Read the model definition and answer for the solid it produces. Units are mm, in the model's axes. A direction names the side the tool comes from. Round coordinates to 2 decimals unless told otherwise and drop trailing zeros. Write each loop counter-clockwise with the first axis right and the second up, starting at its lowest first coordinate (ties: lowest second). Pieces come first, ordered by that corner, then holes. Notation, with made-up numbers: (24, 0.25) - (37, 0.25) arc R36 cw to (37, 39.25) - close; hole circle Ø5 at (-27.75, -7). An arc over 180 degrees is marked (long way). Use one line per item in the form item = value. Start each with the question number.
1) The part is cut by section D-D, the plane y = 16.5. Give the vertices of the cut face in (x, z).
2) For a pull along Z with two mould halves and no side action, classify faces 4 (the face through (46, 22, -58)), 5 (the face through (0, 22, -29)), 6 (the face through (66, 32, -10)) as released by +Z, released by -Z, zero draft, split by the parting line, or undercut.
3) The part is cut by section B-B, the plane x = 17. Give the vertices of the cut face in (y, z), plus the area to 3 significant figures.
4) The part is cut by section C-C, the plane y = 4.5. Count the separate pieces of the cut face and the enclosed holes in it, plus the area to 3 significant figures.
5) Consider line 1 along X through (y, z) = (9, -31); line 2 along Z through (x, y) = (49, 12.5); line 3 along X through (y, z) = (13, -33). Determine where each line is inside the solid, lowest interval first. Write a range as from..to.
6) Each of these flat-tipped pins is pushed along its axis until it touches: pin 1 (1.2 mm diameter, centred on x = 67, z = -51.5, fed in from +Y); pin 2 (10 mm diameter, centred on y = 13, z = -51, fed in from -X); pin 3 (2 mm diameter, centred on x = 39, z = -0.5, fed in from +Y); pin 4 (0.6 mm diameter, centred on x = 37, y = 43.5, fed in from +Z). Where does it stop, or does it pass through?
7) The part is cut by section A-A, the plane y = 33. Give the vertices of the cut face in (x, z).
8) For faces 1 (the face through (72, 42, -1)), 2 (the face through (39.714, 16.79, -9.945)), 3 (the face through (94, 22, -29)), determine the directions among +Z, -Z, +X, -X, +Y, -Y from which every point of the face is accessible in a straight line to the end or side of a thin tool.
from build123d import *

# Parameters (mm, degrees)
SKETCH1_W           = 94
SKETCH1_H           = 58
BOSS_EXTRUDE1_DEPTH = 45
SKETCH2_W           = 90
SKETCH2_H           = 54
CUT_EXTRUDE1_DEPTH  = 43
SKETCH6_W           = 92
SKETCH6_H           = 56
CUT_EXTRUDE2_DEPTH  = 2
SKETCH10_R          = 2
SKETCH10_R_2        = 5.056057686
BOSS_EXTRUDE2_DEPTH = 30
SKETCH11_R          = 3.75
CUT_EXTRUDE3_DEPTH  = 2
SKETCH12_W          = 15.1
SKETCH12_H          = 2
CUT_EXTRUDE4_DEPTH  = 11


with BuildPart() as part:
    # Sketch1 → Boss-Extrude1 (new body)
    with BuildSketch(Plane(origin=(0, 0, 0), x_dir=(1, 0, 0), z_dir=(0, 1, 0))):
        with Locations((47, 29)):
            Rectangle(SKETCH1_W, SKETCH1_H)
    extrude(amount=BOSS_EXTRUDE1_DEPTH)

    # Sketch2 → Cut-Extrude1 (cut)
    with BuildSketch(Plane(origin=(0, 45, 0), x_dir=(1, 0, 0), z_dir=(0, 1, 0))):
        with Locations((47, 29)):
            Rectangle(SKETCH2_W, SKETCH2_H)
    extrude(amount=-CUT_EXTRUDE1_DEPTH, mode=Mode.SUBTRACT)

    # Sketch6 → Cut-Extrude2 (cut)
    with BuildSketch(Plane(origin=(0, 43, 0), x_dir=(-1, 0, 0), z_dir=(0, -1, 0))):
        with Locations((-47, 29)):
            Rectangle(SKETCH6_W, SKETCH6_H)
    extrude(amount=CUT_EXTRUDE2_DEPTH, mode=Mode.SUBTRACT)

    # Sketch10 → Boss-Extrude2 (add)
    with BuildSketch(Plane(origin=(0, 2, 0), x_dir=(1, 0, 0), z_dir=(0, 1, 0))):
        with Locations(Location((6, 50.5, 0), (0, 0, 90))):
            Circle(SKETCH10_R)
        with Locations(Location((66, 50.5, 0), (0, 0, 90))):
            Circle(SKETCH10_R)
        with Locations(Location((6, 10.5, 0), (0, 0, 90))):
            Circle(SKETCH10_R)
        with Locations(Location((66, 10.5, 0), (0, 0, 90))):
            Circle(SKETCH10_R)
        with Locations(Location((37.761829649, 50.378957989, 0), (0, 0, 90))):
            Circle(SKETCH10_R)
        with Locations(Location((37.761829649, 10.378957989, 0), (0, 0, 90))):
            Circle(SKETCH10_R)
        with Locations(Location((37.761829649, 31.073572918, 0), (0, 0, 90))):
            Circle(SKETCH10_R_2)
    extrude(amount=BOSS_EXTRUDE2_DEPTH)

    # Sketch11 → Cut-Extrude3 (cut)
    with BuildSketch(Plane.XY):
        with Locations((19.755158367, 18.08373087)):
            Circle(SKETCH11_R)
    extrude(amount=-CUT_EXTRUDE3_DEPTH, mode=Mode.SUBTRACT)

    # Sketch12 → Cut-Extrude4 (cut)
    with BuildSketch(Plane(origin=(0, 45, 0), x_dir=(1, 0, 0), z_dir=(0, 1, 0))):
        with Locations((42.55, 1)):
            Rectangle(SKETCH12_W, SKETCH12_H)
    extrude(amount=-CUT_EXTRUDE4_DEPTH, mode=Mode.SUBTRACT)


solid = part.part
Geometry results:
q1.outline = (0, -58) - (94, -58) - (94, 0) - (23.15, 0) - (23.15, -2) - (92, -2) - (92, -56) - (2, -56) - (2, -2) - (16.36, -2) - (16.36, 0) - (0, 0) - close; circle Ø4 at (6, -50.5); circle Ø4 at (6, -10.5); circle Ø10.11 at (37.76, -31.07); circle Ø4 at (37.76, -50.38); circle Ø4 at (37.76, -10.38); circle Ø4 at (66, -50.5); circle Ø4 at (66, -10.5)
q2.face_4 = released by -Z
q2.face_5 = zero draft
q2.face_6 = undercut
q3.outline = (0, -58) - (45, -58) - (45, -56) - (43, -56) - (43, -57) - (41, -57) - (41, -56) - (2, -56) - (2, -2) - (15.54, -2) - (15.54, 0) - (0, 0) - close; (20.63, -2) - (41, -2) - (41, -1) - (43, -1) - (43, -2) - (45, -2) - (45, 0) - (20.63, 0) - close
q3.area = 274 mm2
q4.separate_pieces = 8
q4.enclosed_holes = 1
q4.area = 748 mm2
q5.line_1 = 0..2, 32.71..42.82, 92..94
q5.line_2 = -58..-56, -2..0
q5.line_3 = 0..2, 33.09..42.44, 92..94
q6.pin_1 = 32
q6.pin_2 = 0
q6.pin_3 = 34
q6.pin_4 = -56
q7.outline = (0, -58) - (94, -58) - (94, 0) - (0, 0) - close; hole (2, -56) - (92, -56) - (92, -2) - (2, -2) - close
q8.face_1 = none
q8.face_2 = +Y
q8.face_3 = +Z, -Z, +X, +Y, -Y
